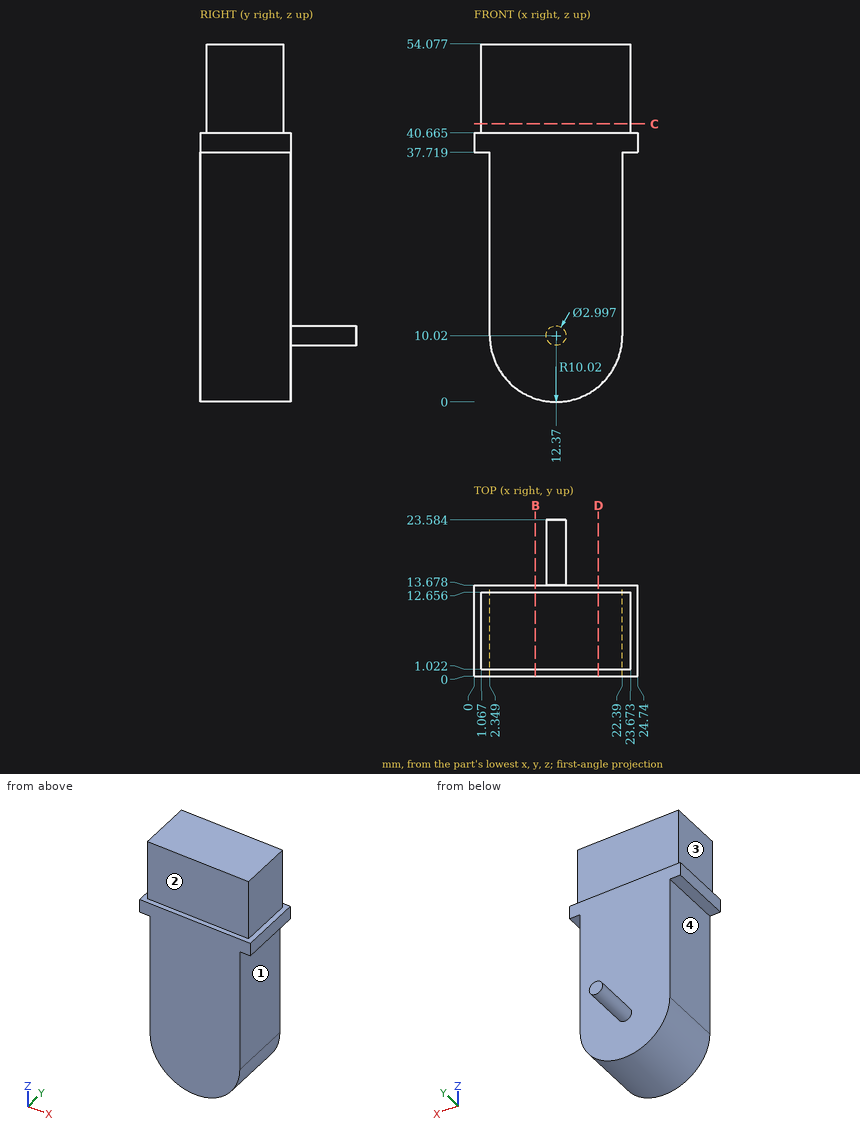
Could you check a few things on this drawing? It's one solid part, dimensions in mm from its lowest x, y, z. A direction names the side the tool comes from. Coordinates: 2 decimals unless noted, no trailing zeros. Write each loop counter-clockwise with the first axis right and the second up, starting at its lowest first coordinate (ties: lowest second). Pieces come first, ordered by that corner, then holes.
Q1. For P1, Ø12.5, axis at x = 12, z = 20.5, coming from the +Y side; P2, Ø4, axis at x = 18, z = 47, coming from the +Y side; P3, Ø7, axis at y = 5, z = 29, coming from the +X side, each with a flat end and sliding along its axis, tell me the tip position at first contact or that it passes through.
Results found:
P1: stops at y = 13.68
P2: stops at y = 12.66
P3: stops at x = 22.39
Q2. Which directions (+Z, -Z, +X, -X, +Y, -Y) give clear straight access to the entire face, cutting with the end or side of a thin tool? Please do the marked faces 1, 2, 3 and 4.
Results found:
face 1: -Z, +X, +Y, -Y
face 2: +Z, +X, -X, -Y
face 3: +Z, -X, +Y, -Y
face 4: -Z, -X, +Y, -Y
Q3. Imagine slicing it at B-B, the plane x = 9.25. List the corners of the cut face in (y, z) for me (1 decimal).
Results found:
outline: (0, 0.5) - (13.7, 0.5) - (13.7, 40.7) - (12.7, 40.7) - (12.7, 54.1) - (1, 54.1) - (1, 40.7) - (0, 40.7) - close
Q4. Please list where these lines run through material, in increasing order: L1, parallel to Y at x = 19, z = 20; L2, parallel to X at y = 1.75, z = 46; L3, parallel to X at y = 2.75, z = 15.
Results found:
L1: y = 0 to 13.68
L2: x = 1.07 to 23.67
L3: x = 2.35 to 22.39
Q5. Imagine slicing it at C-C, the plane z = 42. List the corners of the cut face in (x, y) for me (1 decimal).
Results found:
outline: (1.1, 1) - (23.7, 1) - (23.7, 12.7) - (1.1, 12.7) - close
Q6. Imagine slicing it at D-D, the plane x = 18.75. List the corners of the cut face in (y, z) for me (1 decimal).
Results found:
outline: (0, 2.3) - (13.7, 2.3) - (13.7, 40.7) - (12.7, 40.7) - (12.7, 54.1) - (1, 54.1) - (1, 40.7) - (0, 40.7) - close
